Could you check a few things on this model? Use its own coordinates, in mm. A direction names the side the tool comes from. Coordinates: 2 decimals unless noted, no trailing zeros. Write each loop counter-clockwise with the first axis right and the second up, starting at its lowest first coordinate (ties: lowest second). Pieces come first, ordered by that corner, then holes.
```python
from build123d import *

# Parameters (mm, degrees)
F3_DEPTH = 4.7
F4_R     = 1.116349
F5_DEPTH = 5


with BuildPart() as f1:
    # F0 (on Front) → F1 (revolve)
    with BuildSketch(Plane.XZ):
        Polygon((0, 0), (0, 6), (-7.75, 6), (-7.75, 5.2), (-13.5, 5.2), (-18.7, 0), align=None)
    revolve(axis=Axis((-9.35, 0, 0), (1, 0, 0)))

    # F2 (on face) → F3 (join)
    with BuildSketch(Plane.YZ):
        Polygon((-5.484828, -9.5), (5.484828, -9.5), (10.969655, 0), (5.484828, 9.5), (-5.484828, 9.5), (-10.969655, 0), align=None)
    extrude(amount=F3_DEPTH)

    # F4 (on face) → F5 (join)
    with BuildSketch(Plane.YZ.offset(4.7)):
        with Locations((-2.778471, 0)):
            Circle(F4_R)
        with Locations((2.778471, 0)):
            Circle(F4_R)
        Circle(F4_R)
    extrude(amount=F5_DEPTH)


solid = f1.part
```
1. On a 3-axis mill with a long thin cutter (end or side, diameter ignored), from which of +Z, -Z, +X, -X, +Y, -Y can I reach the whole of each face in a straight line? I mean faces 1 (the face through (2.317, 8.266, 4.684)), 2 (the face through (7.16, 3.38, 0.94)), 3 (the face through (0, 5, 4)). Say none if no direction works.
Verdict:
face 1: +Z, +X, -X, +Y
face 2: +X
face 3: -X
2. If we mould it in two halves opening along Y, with no side actions, what happens to faces 4 (the face through (7.165, -3.894, 0.049)), 5 (the face through (7.16, 0.6, 0.94)), 6 (the face through (9.7, -3, 0)), 7 (the face through (-17.292, 1.375, -0.305))? For each: pulls with the +Y half, pulls with the -Y half, needs draft (parallel to the pull), parting line crosses it, or undercut.
Verdict:
face 4: undercut
face 5: undercut
face 6: needs draft
face 7: parting line crosses it
3. I want a section at D-D on x = -11.5. Please give me the cut outline in (y, z).
Verdict:
outline: circle Ø10.4 at (0, 0)
4. Please list where these lines run through material, in increasing order: line 1 along X through (y, z) = (-4.25, -3.25); line 2 along X through (y, z) = (-7.5, 1.25); line 3 along Y through (x, z) = (4, -2.75).
Verdict:
line 1: x = -7.75 to 4.7
line 2: x = 0 to 4.7
line 3: y = -9.38 to 9.38
5. For pin 1 (12 mm diameter, centred on x = 2.5, y = 7.5, fed in from +Z); pin 2 (4 mm diameter, centred on x = 3, z = -6.5, fed in from +Y); pin 3 (2 mm diameter, centred on y = -4, z = 4.5, fed in from +X); pin 4 (1 mm diameter, centred on x = -1, z = 0.5, fed in from -Y), each with a flat end and sliding along its axis, tell me the tip position at first contact or that it passes through.
Verdict:
pin 1: stops at z = 9.5
pin 2: stops at y = 8.37
pin 3: stops at x = 4.7
pin 4: stops at y = -6
6. I want a section at A-A on x = 4. Please give me the cut outline in (y, z), plus the area to 3 significant figures.
Verdict:
outline: (-10.97, 0) - (-5.48, -9.5) - (5.48, -9.5) - (10.97, 0) - (5.48, 9.5) - (-5.48, 9.5) - close
area: 313 mm2
7. I want a section at C-C on y = 7.75. Please give me the cut outline in (x, z).
Verdict:
outline: (0, -5.58) - (4.7, -5.58) - (4.7, 5.58) - (0, 5.58) - close
8. I want a section at B-B on x = -6. Please give me the cut outline in (y, z).
Verdict:
outline: circle Ø12 at (0, 0)
